Here's how the part is built. I have some questions about the finished solid (model axes, mm). A direction names the side the tool comes from. Coordinates: 2 decimals unless noted, no trailing zeros. Loops run counter-clockwise (first coordinate to the right, second up) from the corner with the lowest first, then second, coordinate; pieces in that order, holes last. Notation, with made-up numbers: M 52.5,1.25 L 98.5,1.25 A26 ccw 98.5,16.25 Z; hole C 66,58.25 d2. An arc over 180 degrees is marked long. Use one line per item in the form item = value. Start each with the question number.
(1) Please list where these lines run through material, in increasing order: L1, parallel to Y at x = 22, z = 1.5; L2, parallel to Y at x = 31.5, z = 8.75; L3, parallel to X at y = -22.5, z = 11.75.
(2) Will these pins go through, and if not, where does the flat tip stop? P1, Ø12, axis at x = 35.5, y = -21.5, coming from the +Z side; P2, Ø4, axis at x = 58.5, z = 8, coming from the -Y side; P3, Ø6, axis at x = 8, z = 11, coming from the +Y side; P4, Ø5.5, axis at x = 65, z = 20, coming from the -Y side.
(3) Imagine slicing it at C-C, the plane y = -41.75. Please give me the cut outline in (x, z), and give its area (3 significant figures).
(4) Thinking about a two-plate mould opening in Z: for faces 4 (the flat face through (58, -50, 5)), 5 (the flat face through (62.5, -20, 13)), 6 (the cylindrical face through (2.47, -40.1, 15.07)), which applies, +Z half, -Z half, draft (parallel to the pull), parting line (faces both ways), or undercut?
(5) Imagine slicing it at D-D, the plane z = 8. State how many separate pieces and enclosed holes the cut face has, and give its area (3 significant figures).
(6) On a 3-axis mill with a long thin cutter (end or side, diameter ignored), from which of +Z, -Z, +X, -X, +Y, -Y can I reach the whole of each face in a straight line? I mean faces 1 (the cylindrical face through (48.4, -2.47, 15.07)), 2 (the flat face through (44, -45, 6)), 3 (the cylindrical face through (30.1, -54.96, 24.14)). Say none if no direction works.
```python
from build123d import *

# Parameters (mm, degrees)
SKETCH_R        = 2
PAD_DEPTH       = 25
SKETCH001_W     = 18.5
SKETCH001_H     = 18.5
POCKET_DEPTH    = 20
CHAMFER_SIZE    = 10
POCKET001_DEPTH = 57.501
POCKET002_DEPTH = 67.501
POCKET003_DEPTH = 25.001
SKETCH005_R     = 1.65
POCKET004_DEPTH = 67.501
SKETCH006_R     = 1.65
POCKET005_DEPTH = 57.501
SKETCH007_W     = 36.5
SKETCH007_H     = 31.5
POCKET006_DEPTH = 12.5
SKETCH008_W     = 5
SKETCH008_H     = 2.222222
POCKET007_DEPTH = 12.5
FILLET_R        = 3
FILLET001_R     = 3
FILLET002_R     = 1
CHAMFER001_SIZE = 0.4
SKETCH009_W     = 10.75
SKETCH009_H     = 5.8
PAD001_DEPTH    = 1
SKETCH010_W     = 15.75
SKETCH010_H     = 5.8
PAD002_DEPTH    = 1
CHAMFER002_SIZE = 0.99


with BuildPart() as part:
    # Sketch → Pad (new body)
    with BuildSketch(Plane.XY):
        Polygon((0, -26), (26, -26), (26, 0), (67.5, 0), (67.5, -57.5), (0, -57.5), align=None)
        with Locations((57.5, -47.5)):
            Circle(SKETCH_R, mode=Mode.SUBTRACT)
    extrude(amount=PAD_DEPTH)

    # Sketch001 (on Face9 of Pad) → Pocket (cut)
    with BuildSketch(Plane.XY.offset(25)):
        with Locations((58.25, -48.25)):
            Rectangle(SKETCH001_W, SKETCH001_H)
    extrude(amount=-POCKET_DEPTH, mode=Mode.SUBTRACT)

    # Chamfer
    chamfer_edges = [part.edges().sort_by_distance(p)[0] for p in [
        (67.5, -57.5, 2.5),
    ]]
    chamfer(chamfer_edges, length=CHAMFER_SIZE)

    # Sketch002 (on Face5 of Chamfer) → Pocket001 (cut, through all)
    with BuildSketch(Plane.XZ.offset(57.5)):
        Polygon((0, 5), (3, 0), (0, 0), align=None)
    extrude(amount=-POCKET001_DEPTH, mode=Mode.SUBTRACT)

    # Sketch003 (on Face2 of Pocket001) → Pocket002 (cut, through all)
    with BuildSketch(Plane.YZ.offset(67.5)):
        Polygon((0, 5), (-3, 0), (0, 0), align=None)
    extrude(amount=-POCKET002_DEPTH, mode=Mode.SUBTRACT)

    # Sketch004 (on Face11 of Pocket002) → Pocket003 (cut, through all)
    with BuildSketch(Plane.XY.offset(25)):
        Polygon((5, -31), (5, -52.5), (44, -52.5), (44, -39), (26, -31), align=None)
        Polygon((31, -26), (49, -34), (62.5, -34), (62.5, -5), (31, -5), align=None)
    extrude(amount=-POCKET003_DEPTH, mode=Mode.SUBTRACT)

    # Sketch005 (on Face24 of Pocket003) → Pocket004 (cut, through all)
    with BuildSketch(Plane(origin=(0, 0, 0), x_dir=(0, -1, 0), z_dir=(-1, 0, 0))):
        with Locations((41.75, 15)):
            Circle(SKETCH005_R)
    extrude(amount=-POCKET004_DEPTH, mode=Mode.SUBTRACT)

    # Sketch006 (on Face20 of Pocket004) → Pocket005 (cut, through all)
    with BuildSketch(Plane(origin=(0, 0, 0), x_dir=(-1, 0, 0), z_dir=(0, 1, 0))):
        with Locations((-46.75, 15)):
            Circle(SKETCH006_R)
    extrude(amount=-POCKET005_DEPTH, mode=Mode.SUBTRACT)

    # Sketch007 (on Face23 of Pocket005) → Pocket006 (cut)
    with BuildSketch(Plane.XY.offset(25)):
        with Locations((49.25, -41.75)):
            Rectangle(SKETCH007_W, SKETCH007_H)
    extrude(amount=-POCKET006_DEPTH, mode=Mode.SUBTRACT)

    # Sketch008 (on Face25 of Pocket006) → Pocket007 (cut)
    with BuildSketch(Plane.XY.offset(25)):
        with Locations((28.5, -32.111111)):
            Rectangle(SKETCH008_W, SKETCH008_H)
    extrude(amount=-POCKET007_DEPTH, mode=Mode.SUBTRACT)

    # Fillet
    fillet_edges = [part.edges().sort_by_distance(p)[0] for p in [
        (31, -55, 25),
        (65, -26, 25),
        (31, -55, 12.5),
        (65, -26, 12.5),
    ]]
    fillet(fillet_edges, radius=FILLET_R)

    # Fillet001
    fillet001_edges = [part.edges().sort_by_distance(p)[0] for p in [
        (5, -52.5, 12.5),
        (5, -31, 12.5),
        (31, -5, 12.5),
        (62.5, -5, 12.5),
        (62.5, -34, 6.25),
        (49, -34, 6.25),
        (44, -39, 6.25),
        (44, -52.5, 6.25),
        (31, -31, 18.75),
        (26, -26, 12.5),
    ]]
    fillet(fillet001_edges, radius=FILLET001_R)

    # Fillet002
    fillet002_edges = [part.edges().sort_by_distance(p)[0] for p in [
        (49, -57.5, 8.75),
        (49, -39, 8.75),
        (67.5, -39, 8.75),
    ]]
    fillet(fillet002_edges, radius=FILLET002_R)

    # Chamfer001
    chamfer001_edges = [part.edges().sort_by_distance(p)[0] for p in [
        (55.5, -47.5, 0),
        (48.4, 0, 15),
        (48.4, -5, 15),
        (5, -40.1, 15),
        (0, -40.1, 15),
    ]]
    chamfer(chamfer001_edges, length=CHAMFER001_SIZE)

    # Sketch009 (on Face32 of Chamfer001) → Pad001 (join)
    with BuildSketch(Plane(origin=(0, 0, 0), x_dir=(0, -1, 0), z_dir=(-1, 0, 0))):
        with Locations((31.375, 15)):
            Rectangle(SKETCH009_W, SKETCH009_H)
        with Locations((52.125, 15)):
            Rectangle(SKETCH009_W, SKETCH009_H)
    extrude(amount=PAD001_DEPTH)

    # Sketch010 (on Face31 of Pad001) → Pad002 (join)
    with BuildSketch(Plane(origin=(0, 0, 0), x_dir=(-1, 0, 0), z_dir=(0, 1, 0))):
        with Locations((-59.625, 15)):
            Rectangle(SKETCH010_W, SKETCH010_H)
        with Locations((-33.875, 15)):
            Rectangle(SKETCH010_W, SKETCH010_H)
    extrude(amount=PAD002_DEPTH)

    # Chamfer002
    chamfer002_edges = [part.edges().sort_by_distance(p)[0] for p in [
        (59.625, 1, 12.1),
        (33.875, 1, 12.1),
        (-1, -31.375, 12.1),
        (-1, -52.125, 12.1),
    ]]
    chamfer(chamfer002_edges, length=CHAMFER002_SIZE)


solid = part.part
```
Answer:
q1.L1 = -57.5 to -52.5, -31 to -26
q1.L2 = -57.5 to -52.5, -33.44 to -26.22, -6.34 to 0
q1.L3 = 26 to 31, 62.5 to 67.5
q2.P1 = 25
q2.P2 = -39
q2.P3 = -26
q2.P4 = -26
q3.outline = M 0,5 L 3,0 L 5,0 L 5,12.95 L 4.6,13.35 L 0.4,13.35 L 0,12.95 Z; M 0,17.05 L 0.4,16.65 L 4.6,16.65 L 5,17.05 L 5,25 L 0,25 Z; M 44,0 L 67.5,0 L 67.5,5 L 49,5 L 49,12.5 L 44,12.5 Z
q3.area = 256 mm²
q4.face_4 = +Z half
q4.face_5 = draft
q4.face_6 = undercut
q5.separate_pieces = 1
q5.enclosed_holes = 2
q5.area = 1,270 mm²
q6.face_1 = +Y, -Y
q6.face_2 = +Z, -Z
q6.face_3 = +Z, +X, -Y
